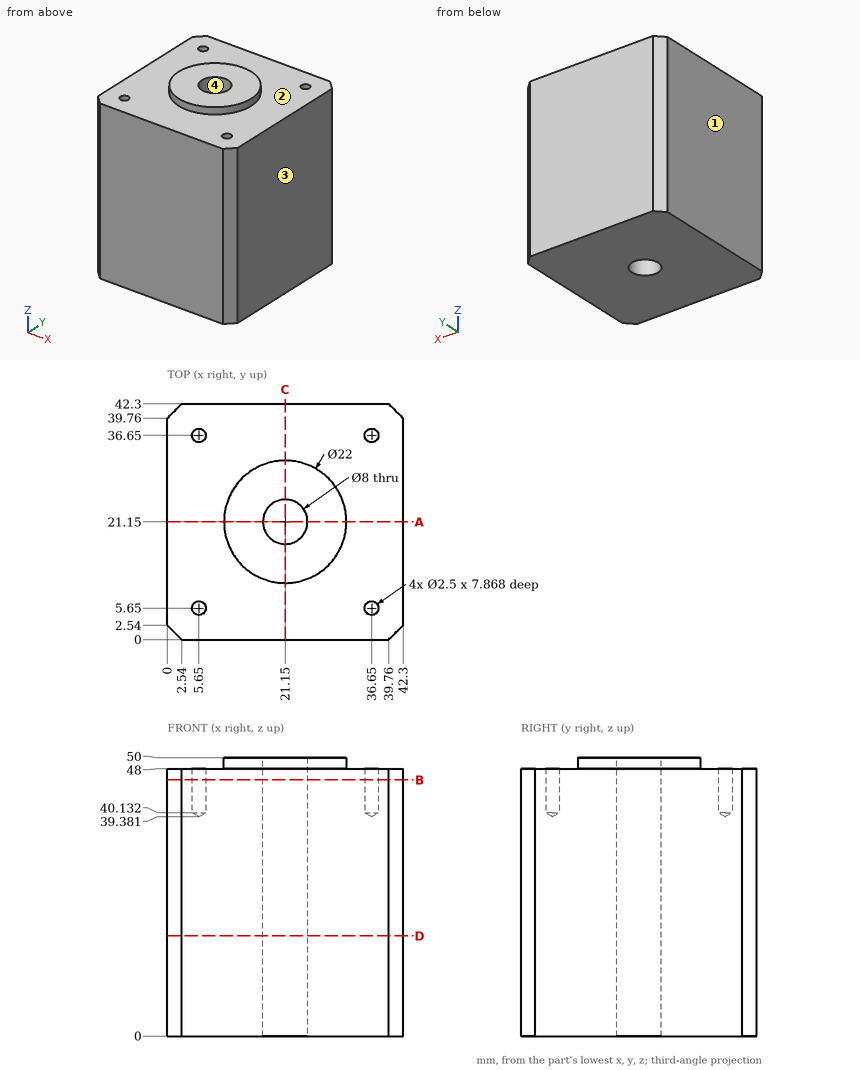
Design review of the part shown in the three views and the two pictorial views. Dimensions are in mm from the part's minimum x, y and z. Give positions to 0.01 mm unless a question says otherwise; leave off trailing zeros. Loops run counter-clockwise (first coordinate to the right, second up) from the corner with the lowest first, then second, coordinate; pieces in that order, holes last. Notation, with made-up numbers: (7.5, 76) -> (17.5, 76) arc R23 ccw to (17.5, 108) -> close; hole circle Ø9 at (-7.75, 14). An arc over 180 degrees is marked (long way). Write each question's results on one line, items separated by ' | '.
1) Take a section at D-D, the plane z = 18. Give the boundary of the cut face in (x, y).
Conclusion:
outline: (0, 2.54) -> (2.54, 0) -> (39.76, 0) -> (42.3, 2.54) -> (42.3, 39.76) -> (39.76, 42.3) -> (2.54, 42.3) -> (0, 39.76) -> close; hole circle Ø8 at (21.15, 21.15)
2) Take a section at A-A, the plane y = 21.15. Give the boundary of the cut face in (x, z), plus the area to 3 significant figures.
Conclusion:
outline: (0, 0) -> (17.15, 0) -> (17.15, 50) -> (10.15, 50) -> (10.15, 48) -> (0, 48) -> close; (25.15, 0) -> (42.3, 0) -> (42.3, 48) -> (32.15, 48) -> (32.15, 50) -> (25.15, 50) -> close | area: 1,670 mm^2
3) For line 1 along X through (y, z) = (36.65, 43.5); line 2 along X through (y, z) = (36, 42), list the stretches that pass through material, from the lowest coordinate up. Write a range as from..to.
Conclusion:
line 1: x = 0..4.4, 6.9..35.4, 37.9..42.3 | line 2: x = 0..4.58, 6.72..35.58, 37.72..42.3
4) Draft analysis for pull direction X (two halves, no side actions). For the marked faces 1, 2, 3 and 4, state which applies: pulls with the +X half, pulls with the -X half, needs draft (parallel to the pull), parting line crosses it, or undercut.
Conclusion:
face 1: pulls with the -X half | face 2: needs draft | face 3: pulls with the +X half | face 4: undercut
5) Insertion check: pin 1 Ø6 at (x, y) = (27.5, 12) entering from +Z; pin 2 Ø3 at (x, y) = (36.65, 36.65) entering from +Z. Each pin has a flat end and moves straight along its axis. Give the tip position at first contact, or say it passes through.
Conclusion:
pin 1: stops at z = 50 | pin 2: stops at z = 48
6) Take a section at B-B, the plane z = 46. Give the boundary of the cut face in (x, y).
Conclusion:
outline: (0, 2.54) -> (2.54, 0) -> (39.76, 0) -> (42.3, 2.54) -> (42.3, 39.76) -> (39.76, 42.3) -> (2.54, 42.3) -> (0, 39.76) -> close; hole circle Ø2.5 at (5.65, 5.65); hole circle Ø2.5 at (5.65, 36.65); hole circle Ø8 at (21.15, 21.15); hole circle Ø2.5 at (36.65, 5.65); hole circle Ø2.5 at (36.65, 36.65)
